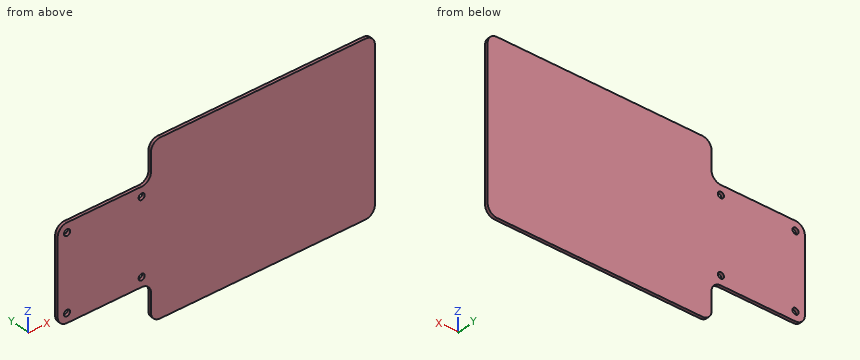
from build123d import *

# Parameters (mm, degrees)
BOSS_EXTRUDE1_DEPTH = 1.6
FILLET1_R           = 5
SKETCH2_R           = 1.65
CUT_EXTRUDE1_DEPTH  = 152.830695184


with BuildPart() as part:
    # Sketch1 → Boss-Extrude1 (new body)
    with BuildSketch(Plane(origin=(0, 0, 0), x_dir=(1, 0, 0), z_dir=(0, 1, 0))):
        Polygon((-25, 25), (25, 25), (25, 45), (145, 45), (145, -45), (25, -45), (25, -25), (-25, -25), align=None)
    extrude(amount=BOSS_EXTRUDE1_DEPTH)

    # Fillet1
    fillet1_edges = [part.edges().sort_by_distance(p)[0] for p in [
        (-25, 0.8, 25),
        (-25, 0.8, -25),
        (25, 0.8, -25),
        (25, 0.8, -45),
        (145, 0.8, -45),
        (145, 0.8, 45),
        (25, 0.8, 45),
        (25, 0.8, 25),
    ]]
    fillet(fillet1_edges, radius=FILLET1_R)

    # Sketch2 → Cut-Extrude1 (cut, through all)
    with BuildSketch(Plane(origin=(0, 1.6, 0), x_dir=(1, 0, 0), z_dir=(0, 1, 0))):
        with Locations(Location((-20, 20, 0), (0, 0, 270))):
            Circle(SKETCH2_R)
        with Locations(Location((20, 20, 0), (0, 0, 270))):
            Circle(SKETCH2_R)
        with Locations(Location((20, -20, 0), (0, 0, 270))):
            Circle(SKETCH2_R)
        with Locations(Location((-20, -20, 0), (0, 0, 270))):
            Circle(SKETCH2_R)
    extrude(amount=-CUT_EXTRUDE1_DEPTH, mode=Mode.SUBTRACT)


solid = part.part
Input: part model. Units: mm. Frame: model coordinates. Coordinates: 2 decimals unless noted, no trailing zeros. Loops run counter-clockwise (first coordinate to the right, second up) from the corner with the lowest first, then second, coordinate; pieces in that order, holes last.
Q1. Cut plane A-A (y = 0.8). Output: boundary loops of the cut face in (x, z), then the cut area to 3 significant figures.
Q2. Contact query for flat-ended pins moving along their axis: pin 1 (0.5 mm diameter, centred on x = 3.5, y = 1, fed in from -Z); pin 2 (0.8 mm diameter, centred on y = 1, z = -36.5, fed in from -X). Output: stop coordinate, or through.
Q3. Cut plane B-B (z = -37). Output: boundary loops of the cut face in (x, y).
Q4. Cut plane C-C (x = -10). Output: boundary loops of the cut face in (y, z), then the cut area to 3 significant figures.
Q5. Material intervals for line 1 (X direction, y = 0.7, z = -20); line 2 (X direction, y = 0.65, z = 31); line 3 (Z direction, x = -8, y = 1.3), sorted ascending.
Working result:
1. outline: (-25, -20) arc R5 ccw to (-20, -25) - (20, -25) arc R5 cw to (25, -30) - (25, -40) arc R5 ccw to (30, -45) - (140, -45) arc R5 ccw to (145, -40) - (145, 40) arc R5 ccw to (140, 45) - (30, 45) arc R5 ccw to (25, 40) - (25, 30) arc R5 cw to (20, 25) - (-20, 25) arc R5 ccw to (-25, 20) - close; hole circle Ø3.3 at (-20, -20); hole circle Ø3.3 at (-20, 20); hole circle Ø3.3 at (20, -20); hole circle Ø3.3 at (20, 20)
1. area: 13,200 mm2
2. pin 1: stops at z = -25
2. pin 2: stops at x = 25
3. outline: (25, 0) - (145, 0) - (145, 1.6) - (25, 1.6) - close
4. outline: (0, -25) - (1.6, -25) - (1.6, 25) - (0, 25) - close
4. area: 80.0 mm2
5. line 1: x = -25 to -21.65, -18.35 to 18.35, 21.65 to 145
5. line 2: x = 25 to 145
5. line 3: z = -25 to 25
